Check sheet for the modelled part. Datum: model origin and axes. Units: mm. A direction names the side the tool comes from. Give positions to 0.01 mm unless a question says otherwise; leave off trailing zeros. Loops run counter-clockwise (first coordinate to the right, second up) from the corner with the lowest first, then second, coordinate; pieces in that order, holes last. Notation, with made-up numbers: (-17.5, 21) -> (5.5, 21) arc R18 ccw to (5.5, 39) -> close; hole circle Ø7 at (-15.75, 35). An arc over 180 degrees is marked (long way). Write each question's results on one line, items separated by ' | '. Start each with the question number.
1. Cross-section at A-A on z = -57. Record the boundary of the cut face in (x, y), and give its area (3 significant figures).
2. Gauge pin test, flat ends, axial feed: pin 1 Ø23.5 at (y, z) = (3, -52) entering from -X; pin 2 Ø4.5 at (x, z) = (-16, -53.65) entering from -Y; pin 3 Ø1.5 at (x, z) = (3, -46) entering from -Y. Record the tip position at first contact, or that the pin passes through.
3. Tool access check on faces 5 (the face through (2.46, 19.54, -19.45)), 6 (the face through (2, 21.15, 0)), 7 (the face through (-10, 24.98, -56)), 8 (the face through (2.54, 10.5, -66.09)). Record the directions out of +Z, -Z, +X, -X, +Y, -Y that give a thin tool (end or side, any length) a straight path to the whole face; none if there is none.
4. Cross-section at D-D on x = -10. Record the boundary of the cut face in (y, z), and give its area (3 significant figures).
5. Cross-section at B-B on y = -7. Record the boundary of the cut face in (x, z), and give its area (3 significant figures).
6. Material ranges on L1, parallel to Y at x = 2, z = 15.5 (3 decimals); L2, parallel to Z at x = 1.5, y = 2, recorded low to high. Write a range as from..to.
7. Cross-section at C-C on x = -16. Record the boundary of the cut face in (y, z), and give its area (3 significant figures).
8. Mould release check, pull along Y, two halves, no side actions. Record for faces 1 (the face through (2, 12, -56)), 2 (the face through (-9.1, 26, -70.5)), 3 (the face through (2.46, 16.57, -36.53)), 4 (the face through (2, -21.15, 0)): +Y half, -Y half, draft (parallel to the pull), parting line (faces both ways), or undercut.
from build123d import *

# Parameters (mm, degrees)
SKETCH_1_R          = 10
SKETCH_1_R_2        = 1.475
EXTRUDE_1_DEPTH     = 5
FILLET_1_R          = 5
FILLET_2_R          = 5
FILLET_3_R          = 5
FILLET_4_R          = 5
FILLET_5_R          = 2
SKETCH_4_W          = 30
SKETCH_4_H          = 2.02
EXTRUDE_2_DEPTH     = 20
FILLET_11_R         = 0.5
FILLET_12_R         = 0.5
RIB_5_REACH         = 106.233
SKETCH_5_WALL_W     = 231.251388166
SKETCH_5_WALL_H     = 30
SKETCH_12_W         = 11
SKETCH_12_H         = 10.392304845
CUT_EXTRUDE_1_DEPTH = 20
FILLET_14_R         = 0.5
FILLET_15_R         = 0.5
SKETCH_14_R         = 1.46
CUT_EXTRUDE_2_DEPTH = 44


with BuildPart() as part:
    # 草图1 → 凸台-拉伸1 (new body)
    with BuildSketch(Plane(origin=(0, 0, 0), x_dir=(0, 0, -1), z_dir=(1, 0, 0))):
        with BuildLine():
            ThreePointArc((77.019141235, 27), (77.372694625, 26.853553391), (77.519141235, 26.5))
            Line((77.519141235, 26.5), (77.519141235, -9.130858765))
            Line((77.519141235, -9.130858765), (47.519141235, -9.130858765))
            Line((47.519141235, -9.130858765), (27.519141235, -9.130858765))
            ThreePointArc((27.519141235, -9.130858765), (23.015478277, -10.996337043), (21.15, -15.5))
            ThreePointArc((21.15, -15.5), (19.495153314, -19.495153314), (15.5, -21.15))
            Line((15.5, -21.15), (-15.5, -21.15))
            ThreePointArc((-15.5, -21.15), (-19.495153314, -19.495153314), (-21.15, -15.5))
            Line((-21.15, -15.5), (-21.15, 15.5))
            ThreePointArc((-21.15, 15.5), (-19.495153314, 19.495153314), (-15.5, 21.15))
            Line((-15.5, 21.15), (15.5, 21.15))
            ThreePointArc((15.5, 21.15), (19.495153314, 19.495153314), (21.15, 15.5))
            ThreePointArc((21.15, 15.5), (22.456034545, 11.635946336), (25.838516133, 9.356592205))
            Line((25.838516133, 9.356592205), (47.519141235, 23.98))
            Line((47.519141235, 23.98), (47.519141235, 26.5))
            ThreePointArc((47.519141235, 26.5), (47.665587844, 26.853553391), (48.019141235, 27))
            Line((48.019141235, 27), (77.019141235, 27))
        make_face()
        Circle(SKETCH_1_R, mode=Mode.SUBTRACT)
        with Locations((-15.5, -15.5)):
            Circle(SKETCH_1_R_2, mode=Mode.SUBTRACT)
        with Locations((15.5, -15.5)):
            Circle(SKETCH_1_R_2, mode=Mode.SUBTRACT)
        with Locations((15.5, 15.5)):
            Circle(SKETCH_1_R_2, mode=Mode.SUBTRACT)
        with Locations((-15.5, 15.5)):
            Circle(SKETCH_1_R_2, mode=Mode.SUBTRACT)
        Polygon((53.519141235, 0.869141235), (31.13826194, 0.869141235), (47.640843236, 12), (67.519141235, 12), (67.519141235, 0.869141235), (59.519141235, 0.869141235), align=None, mode=Mode.SUBTRACT)
    extrude(amount=EXTRUDE_1_DEPTH)

    # 圆角1
    fillet_1_edges = [part.edges().sort_by_distance(p)[0] for p in [
        (2.5, -9.130858765, -77.519141235),
    ]]
    fillet(fillet_1_edges, radius=FILLET_1_R)

    # 圆角2
    fillet_2_edges = [part.edges().sort_by_distance(p)[0] for p in [
        (2.5, 12, -67.519141235),
    ]]
    fillet(fillet_2_edges, radius=FILLET_2_R)

    # 圆角3
    fillet_3_edges = [part.edges().sort_by_distance(p)[0] for p in [
        (2.5, 12, -47.640843236),
    ]]
    fillet(fillet_3_edges, radius=FILLET_3_R)

    # 圆角4
    fillet_4_edges = [part.edges().sort_by_distance(p)[0] for p in [
        (2.5, 0.869141235, -67.519141235),
    ]]
    fillet(fillet_4_edges, radius=FILLET_4_R)

    # 圆角5
    fillet_5_edges = [part.edges().sort_by_distance(p)[0] for p in [
        (2.5, 0.869141235, -31.13826194),
    ]]
    fillet(fillet_5_edges, radius=FILLET_5_R)

    # 草图4 → 凸台-拉伸2 (add)
    with BuildSketch(Plane(origin=(0, 0, 0), x_dir=(0, 0, -1), z_dir=(1, 0, 0))):
        with Locations((62.519141235, 25.99)):
            Rectangle(SKETCH_4_W, SKETCH_4_H)
    extrude(amount=-EXTRUDE_2_DEPTH)

    # 圆角11
    fillet_11_edges = [part.edges().sort_by_distance(p)[0] for p in [
        (-10, 27, -47.519141235),
    ]]
    fillet(fillet_11_edges, radius=FILLET_11_R)

    # 圆角12
    fillet_12_edges = [part.edges().sort_by_distance(p)[0] for p in [
        (-10, 27, -77.519141235),
    ]]
    fillet(fillet_12_edges, radius=FILLET_12_R)

    # 草图5 wall → 筋5 (add, up to next)
    with BuildSketch(Plane(origin=(-9, 19.783847578, -77.519141235), x_dir=(-0.866025403793, 0.499999999985, 0), z_dir=(-0.499999999985, -0.866025403793, 0)), mode=Mode.PRIVATE) as rib_5_sk1:
        with Locations((0, -15)):
            Rectangle(SKETCH_5_WALL_W, SKETCH_5_WALL_H)
    rib_5_tool1 = extrude(rib_5_sk1.sketch, amount=-RIB_5_REACH, mode=Mode.PRIVATE) - part.part
    add(rib_5_tool1.solids().sort_by_distance((-9, 19.783847578, -77.519141235))[0])

    # 草图12 → 切除-拉伸1 (cut)
    with BuildSketch(Plane.ZY.offset(20)):
        with Locations((-72.019141235, 19.783847578)):
            Rectangle(SKETCH_12_W, SKETCH_12_H)
        with Locations((-53.019141235, 19.783847578)):
            Rectangle(SKETCH_12_W, SKETCH_12_H)
    extrude(amount=-CUT_EXTRUDE_1_DEPTH, mode=Mode.SUBTRACT)

    # 圆角14
    fillet_14_edges = [part.edges().sort_by_distance(p)[0] for p in [
        (-10, 24.98, -77.519141235),
    ]]
    fillet(fillet_14_edges, radius=FILLET_14_R)

    # 圆角15
    fillet_15_edges = [part.edges().sort_by_distance(p)[0] for p in [
        (-10, 24.98, -47.519141235),
    ]]
    fillet(fillet_15_edges, radius=FILLET_15_R)

    # 草图14 → 切除-拉伸2 (cut)
    with BuildSketch(Plane(origin=(0, 0, 0), x_dir=(1, 0, 0), z_dir=(0, 1, 0))):
        with Locations(Location((-10, 71.650840547, 0), (0, 0, 90))):
            Circle(SKETCH_14_R)
        with Locations(Location((-16, 71.650840547, 0), (0, 0, 90))):
            Circle(SKETCH_14_R)
        with Locations(Location((-10, 53.650840547, 0), (0, 0, 90))):
            Circle(SKETCH_14_R)
        with Locations(Location((-16, 53.650840547, 0), (0, 0, 90))):
            Circle(SKETCH_14_R)
    extrude(amount=CUT_EXTRUDE_2_DEPTH, mode=Mode.SUBTRACT)


solid = part.part
Geometry says:
1) outline: (-20, 24.98) -> (0, 24.98) -> (0, 12) -> (5, 12) -> (5, 27) -> (-20, 27) -> close; (0, -9.13) -> (5, -9.13) -> (5, 0.87) -> (0, 0.87) -> close | area: 165 mm^2
2) pin 1: x = 0 | pin 2: y = 24.98 | pin 3: y = -9.13
3) face 5: +X, -X, +Y | face 6: +Z, +X, -X, +Y | face 7: -X, -Y | face 8: +X, -X
4) outline: (20.36, -66.52) -> (24.98, -66.52) -> (24.98, -70.19) -> (27, -70.19) -> (27, -55.11) -> (24.98, -55.11) -> (24.98, -58.52) -> (20.36, -58.52) -> close; (24.98, -77.02) arc R0.5 ccw to (25.48, -77.52) -> (26.5, -77.52) arc R0.5 ccw to (27, -77.02) -> (27, -73.11) -> (24.98, -73.11) -> close; (24.98, -52.19) -> (27, -52.19) -> (27, -48.02) arc R0.5 ccw to (26.5, -47.52) -> (25.48, -47.52) arc R0.5 ccw to (24.98, -48.02) -> close | area: 85.5 mm^2
5) outline: (0, -76.61) -> (5, -76.61) -> (5, -7.14) -> (0, -7.14) -> close; (0, 7.14) -> (5, 7.14) -> (5, 21.15) -> (0, 21.15) -> close | area: 417 mm^2
6) L1: -21.15..-16.975, -14.025..14.025, 16.975..21.15 | L2: -77.52..-65.69, -35.88..-9.8, 9.8..21.15
7) outline: (23.83, -66.52) -> (24.98, -66.52) -> (24.98, -70.19) -> (27, -70.19) -> (27, -55.11) -> (24.98, -55.11) -> (24.98, -58.52) -> (23.83, -58.52) -> close; (24.98, -77.02) arc R0.5 ccw to (25.48, -77.52) -> (26.5, -77.52) arc R0.5 ccw to (27, -77.02) -> (27, -73.11) -> (24.98, -73.11) -> close; (24.98, -52.19) -> (27, -52.19) -> (27, -48.02) arc R0.5 ccw to (26.5, -47.52) -> (25.48, -47.52) arc R0.5 ccw to (24.98, -48.02) -> close | area: 57.8 mm^2
8) face 1: undercut | face 2: draft | face 3: +Y half | face 4: -Y half
